Build history of the part. All positions in model axes, mm. A direction names the side the tool comes from. Coordinates: 2 decimals unless noted, no trailing zeros. Order: outer loops, then holes, each group sorted by start corner. A loop starts at its lowest first (then second) coordinate and runs counter-clockwise, first axis right, second up. Notation, with made-up numbers: M 3,-18.75 L 19,-18.75 A11 cw 19,-2.75 Z; hole C -4,79.25 d11. An arc over 180 degrees is marked long. Write item = value, one per line. Start each with the question number.
Q1. 3-axis set-ups, long thin cutter, end or side, ignore diameter. For faces 5 (the face through (1, 15, -1)), 6 (the face through (0, 7, 22)): which of +Z, -Z, +X, -X, +Y, -Y reach the whole face in a straight line?
Q2. Pin check, flat tip, straight feed: P1, Ø4.5, axis at x = 3, z = 26, coming from the +Y side. Stop position of the tip, or through.
Q3. Band-saw the part on B-B on z = -27. Write the cut outline in (x, y).
Q4. Pull direction X, two halves, no side cores. Call faces 1 (the face through (1.352, 3.451, 22.708)), 2 (the face through (41.99, 7.4, -42.15)), 3 (the face through (0, 7, 45)), 4 (the face through (0.33, 11.056, -34.493)): released by +X, released by -X, zero draft, split by the parting line, or undercut.
Q5. Band-saw the part on C-C on y = 8.25. Write the cut outline in (x, z), plus the area to 3 significant figures.
Q6. Drill centre lines: probe 1 along X at (y, z) = (5.75, -27); probe 2 along X at (y, z) = (13.25, -27); probe 3 along Z at (x, y) = (-39, 11). Where is each one in solid material? Low to high.
Q7. Band-saw the part on D-D on z = -39. Write the cut outline in (x, y), plus the area to 3 significant figures.
Q8. Band-saw the part on A-A on x = 0. Write the cut outline in (y, z).
```python
from build123d import *

# Parameters (mm, degrees)
EXTRUDE_2_DEPTH     = 15
SKETCH_3_R          = 7.5
CUT_EXTRUDE_1_DEPTH = 8
SKETCH_4_R          = 4.5
CUT_EXTRUDE_2_DEPTH = 66.383484153


with BuildPart() as part:
    # 草图2 → 凸台-拉伸2 (new body)
    with BuildSketch(Plane(origin=(0, 0, 0), x_dir=(1, 0, 0), z_dir=(0, 1, 0))):
        with BuildLine():
            Line((-35, 45), (35, 45))
            ThreePointArc((35, 45), (42.071067812, 42.071067812), (45, 35))
            Line((45, 35), (45, -35))
            ThreePointArc((45, -35), (42.071067812, -42.071067812), (35, -45))
            Line((35, -45), (-35, -45))
            ThreePointArc((-35, -45), (-42.071067812, -42.071067812), (-45, -35))
            Line((-45, -35), (-45, 35))
            ThreePointArc((-45, 35), (-42.071067812, 42.071067812), (-35, 45))
        make_face()
    extrude(amount=EXTRUDE_2_DEPTH)

    # 草图3 → 切除-拉伸1 (cut)
    with BuildSketch(Plane(origin=(0, 15, 0), x_dir=(1, 0, 0), z_dir=(0, 1, 0))):
        with Locations(Location((0, 27, 0), (0, 0, 270))):
            Circle(SKETCH_3_R)
        with Locations(Location((0, -27, 0), (0, 0, 90))):
            Circle(SKETCH_3_R)
    extrude(amount=-CUT_EXTRUDE_1_DEPTH, mode=Mode.SUBTRACT)

    # 草图4 → 切除-拉伸2 (cut, through all)
    with BuildSketch(Plane.XZ):
        with Locations(Location((0, 27, 0), (0, 0, 270))):
            Circle(SKETCH_4_R)
        with Locations(Location((0, -27, 0), (0, 0, 90))):
            Circle(SKETCH_4_R)
    extrude(amount=-CUT_EXTRUDE_2_DEPTH, mode=Mode.SUBTRACT)


solid = part.part
```
Recorded:
q1.face_5 = +Z, -Z, +X, -X, +Y
q1.face_6 = +Y
q2.P1 = 7
q3.outline = M -45,0 L -4.5,0 L -4.5,7 L -7.5,7 L -7.5,15 L -45,15 Z; M 4.5,0 L 45,0 L 45,15 L 7.5,15 L 7.5,7 L 4.5,7 Z
q4.face_1 = undercut
q4.face_2 = released by +X
q4.face_3 = zero draft
q4.face_4 = undercut
q5.outline = M -45,-35 A10 ccw -35,-45 L 35,-45 A10 ccw 45,-35 L 45,35 A10 ccw 35,45 L -35,45 A10 ccw -45,35 Z; hole C 0,-27 d15; hole C 0,27 d15
q5.area = 7,660 mm2
q6.probe_1 = -45 to -4.5, 4.5 to 45
q6.probe_2 = -45 to -7.5, 7.5 to 45
q6.probe_3 = -44.17 to 44.17
q7.outline = M -44.17,0 L 44.17,0 L 44.17,15 L -44.17,15 Z
q7.area = 1,320 mm2
q8.outline = M 0,-45 L 15,-45 L 15,-34.5 L 7,-34.5 L 7,-31.5 L 0,-31.5 Z; M 0,-22.5 L 7,-22.5 L 7,-19.5 L 15,-19.5 L 15,19.5 L 7,19.5 L 7,22.5 L 0,22.5 Z; M 0,31.5 L 7,31.5 L 7,34.5 L 15,34.5 L 15,45 L 0,45 Z
